Design review of the part built by this model. Coordinates are the model's own, in mm. Face numbers are marked on the shaded views. A direction names the side the tool comes from. Give positions to 0.01 mm unless a question says otherwise; leave off trailing zeros. Write each loop counter-clockwise with the first axis right and the second up, starting at its lowest first coordinate (ties: lowest second). Pieces come first, ordered by that corner, then holes. Notation, with made-up numbers: M 43.25,-31.75 L 70.25,-31.75 A23 cw 70.25,7.25 Z; hole C -2,88 d10. An arc over 180 degrees is marked long. Use one line per item in the form item = value. Start each with the question number.
from build123d import *

# Parameters (mm, degrees)
SKETCH_1_R      = 14
SKETCH_1_R_2    = 1.6
SKETCH_1_R_3    = 3
EXTRUDE_2_DEPTH = 4
SKETCH_2_R      = 7.5
SKETCH_2_R_2    = 3
EXTRUDE_3_DEPTH = 12


with BuildPart() as part:
    # ｽｹｯﾁ1 → ﾎﾞｽ - 押し出し2 (new body)
    with BuildSketch(Plane.XY):
        Circle(SKETCH_1_R)
        with Locations((10.5, 0)):
            Circle(SKETCH_1_R_2, mode=Mode.SUBTRACT)
        with Locations((-5.25, 9.09326674)):
            Circle(SKETCH_1_R_2, mode=Mode.SUBTRACT)
        with Locations((-5.25, -9.09326674)):
            Circle(SKETCH_1_R_2, mode=Mode.SUBTRACT)
        Circle(SKETCH_1_R_3, mode=Mode.SUBTRACT)
    extrude(amount=EXTRUDE_2_DEPTH)

    # ｽｹｯﾁ2 → ﾎﾞｽ - 押し出し3 (add)
    with BuildSketch(Plane.XY.offset(4)):
        Circle(SKETCH_2_R)
        Circle(SKETCH_2_R_2, mode=Mode.SUBTRACT)
    extrude(amount=EXTRUDE_3_DEPTH)


solid = part.part
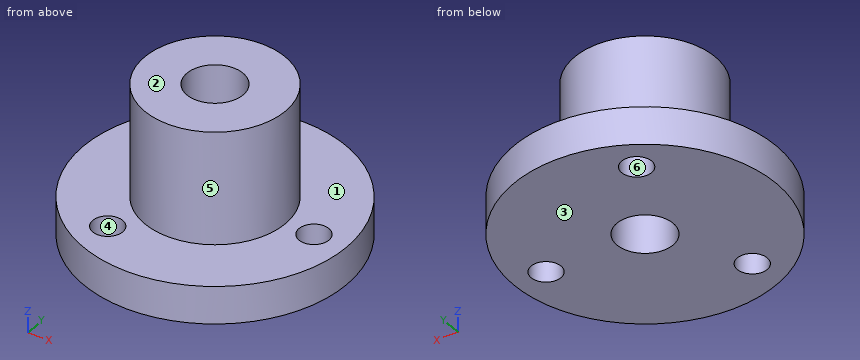
1. We need section A-A (x = 0). State the section outline as (y, z) points, and give its area (3 significant figures).
2. To check wall thickness, follow L1, parallel to Y at x = 0, z = 7.5; L2, parallel to Y at x = -5.25, z = 3.15; L3, parallel to Z at x = 8.25, y = 6. State the ranges of each line that lie inside material, in increasing order.
3. Clearance check with flat-ended pins moving along their axes: pin 1 Ø5 at (x, y) = (-5.25, -9.09) entering from +Z; pin 2 Ø1.5 at (x, z) = (-6.5, 13.5) entering from -Y; pin 3 Ø1.5 at (y, z) = (-10, 13) entering from -X (3 decimals). State where each tip first meets the part, or that it passes through.
4. We need section C-C (x = -5.25). State the section outline as (y, z) points.
5. For the marked faces 1 and 2, list the 3-axis set-ups (+Z, -Z, +X, -X, +Y, -Y) from which the entire face can be reached by the end or side of a thin tool; tool diameter is ignored.
6. We need section B-B (y = 0). State the section outline as (x, z) points.
7. We need section D-D (z = 14.75). State the section outline as (x, y) points.
8. Draft analysis for pull direction X (two halves, no side actions). For the marked faces 3, 4, 5 and 6, state which applies: pulls with the +X half, pulls with the -X half, needs draft (parallel to the pull), parting line crosses it, or undercut.
Answer block:
q1.outline = M -14,0 L -3,0 L -3,16 L -7.5,16 L -7.5,4 L -14,4 Z; M 3,0 L 14,0 L 14,4 L 7.5,4 L 7.5,16 L 3,16 Z
q1.area = 196 mm^2
q2.L1 = -7.5 to -3, 3 to 7.5
q2.L2 = -12.98 to -10.69, -7.49 to 7.49, 10.69 to 12.98
q2.L3 = 0 to 4
q3.pin_1 = 4
q3.pin_2 = -4.82
q3.pin_3 = through
q4.outline = M -12.98,0 L -10.69,0 L -10.69,4 L -12.98,4 Z; M -7.49,0 L 7.49,0 L 7.49,4 L 5.36,4 L 5.36,16 L -5.36,16 L -5.36,4 L -7.49,4 Z; M 10.69,0 L 12.98,0 L 12.98,4 L 10.69,4 Z
q5.face_1 = +Z
q5.face_2 = +Z, +X, -X, +Y, -Y
q6.outline = M -14,0 L -3,0 L -3,16 L -7.5,16 L -7.5,4 L -14,4 Z; M 3,0 L 8.9,0 L 8.9,4 L 7.5,4 L 7.5,16 L 3,16 Z; M 12.1,0 L 14,0 L 14,4 L 12.1,4 Z
q7.outline = C 0,0 d15; hole C 0,0 d6
q8.face_3 = needs draft
q8.face_4 = undercut
q8.face_5 = parting line crosses it
q8.face_6 = undercut
